Part model, mm, in its own coordinate system. Give positions to 0.01 mm unless a question says otherwise; leave off trailing zeros. Order: outer loops, then holes, each group sorted by start corner. A loop starts at its lowest first (then second) coordinate and runs counter-clockwise, first axis right, second up. Notation, with made-up numbers: (47, -3) -> (81, -3) arc R22 ccw to (81, 26) -> close; hole circle Ø7 at (8, 82). An arc over 180 degrees is marked (long way). Write item = value, one per line. Start each with the question number.
Item 1: Band-saw the part on B-B on y = -0.6. Count the separate pieces of the cut face and the enclosed holes in it, plus the area to 3 significant figures.
Item 2: Drill centre lines: line 1 along Z through (x, y) = (10, -0.05); line 2 along X through (y, z) = (-1.15, -3); line 3 along Z through (x, y) = (-7, -0.65). Where is each one in solid material? Low to high.
Item 3: Band-saw the part on A-A on x = -7.19. Write the cut outline in (y, z).
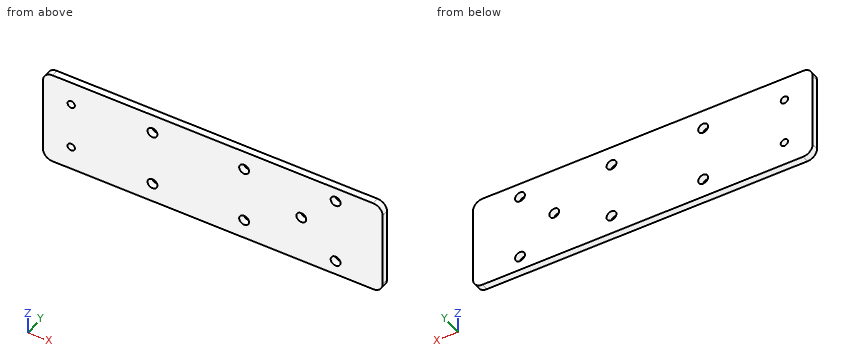
Autodesk Inventor part; units mm, degrees
ref_plane "YZ Plane" through (0, 0, 0) normal (1, 0, 0) x (0, 1, 0)
ref_plane "XZ Plane" through (0, 0, 0) normal (0, 1, 0) x (-1, 0, 0)
ref_plane "XY Plane" through (0, 0, 0) normal (0, 0, 1) x (1, 0, 0)
sketch "Sketch1" plane through (0, 0, 0) normal (0, 1, 0) x (-1, 0, 0)
  line L0 (-0.4496, -20.14) -> (-0.4496, 0)
  circle A0 centre (-29.6093, -16.045) radius 1.05
  circle A1 centre (-29.6093, -4.095) radius 1.05
  circle A2 centre (-10.1093, -4.095) radius 1.05
  circle A3 centre (-10.1093, -16.045) radius 1.05
  circle A4 centre (7.19, -5.07) radius 0.7835
  circle A5 centre (7.19, -15.07) radius 0.7835
  circle A6 centre (-41.7893, -10.07) radius 1.05
  circle A7 centre (-49.0893, -17.07) radius 1.05
  circle A8 centre (-49.0893, -3.07) radius 1.05
  arc A9 (-59.0893, -18.14) -> (-57.0893, -20.14) centre (-57.0893, -18.14) ccw
  line L1 (-59.0893, -2) -> (-59.0893, -18.14)
  arc A10 (-57.0893, 0) -> (-59.0893, -2) centre (-57.0893, -2) ccw
  arc A11 (11.19, -20.14) -> (13.19, -18.14) centre (11.19, -18.14) ccw
  line L2 (13.19, -2) -> (13.19, -18.14)
  arc A12 (13.19, -2) -> (11.19, 0) centre (11.19, -2) ccw
  line L3 (-57.0893, 0) -> (11.19, 0)
  line L4 (11.19, -20.14) -> (-57.0893, -20.14)
  line L5 (-0.8993, -20.14) -> (-0.8993, 0)
  line L6 (0, 0) -> (0, -20.14)
extrude "Plate1" add sketch "Sketch1" against normal blind 1.5
equation "\"d0\" = Thickness"
equation "\"BendReliefWidth\" = Thickness"
equation "\"BendReliefDepth\" = 0.5 * Thickness"
equation "\"CornerReliefSize\" = 4 * Thickness"
equation "\"MinimumRemnant\" = 2 * Thickness"
equation "\"TransitionRadius\" = BendRadius"
equation "\"JacobiRadiusSize\" = BendRadius"
equation "\"GapSize\" = Thickness"
properties part number "CAM_servo_bracket_top" material "Aluminum 6061"
Values found:
q1.separate_pieces = 1
q1.enclosed_holes = 9
q1.area = 1,420 mm^2
q2.line_1 = -20.14 to -17.09, -15 to -5.14, -3.05 to 0
q2.line_2 = -13.19 to 48.04, 50.14 to 59.09
q2.line_3 = -20.14 to -15.83, -14.31 to -5.83, -4.31 to 0
q3.outline = (-1.5, -20.14) -> (0, -20.14) -> (0, -15.85) -> (-1.5, -15.85) -> close; (-1.5, -14.29) -> (0, -14.29) -> (0, -5.85) -> (-1.5, -5.85) -> close; (-1.5, -4.29) -> (0, -4.29) -> (0, 0) -> (-1.5, 0) -> close
